```python
from build123d import *

# Parameters (mm, degrees)
F0_R      = 10
F1_DEPTH  = 20
F1_FACE_W = 40
F1_FACE_H = 40
F2_DEPTH  = 10
F4_DEPTH  = 40.001
F5_R      = 4


with BuildPart() as f1:
    # F0 (on Front) → F1 (new body, symmetric)
    with BuildSketch(Plane.XZ):
        Polygon((-12, 21.5), (-20, 21.5), (-20, -21.5), (20, -21.5), (20, 8), align=None)
        Circle(F0_R, mode=Mode.SUBTRACT)
    extrude(amount=F1_DEPTH, both=True)

    # F1_face (on face) → F2 (join)
    with BuildSketch(Plane(origin=(0, 0, -21.5), x_dir=(1, 0, 0), z_dir=(0, 0, -1))):
        Rectangle(F1_FACE_W, F1_FACE_H)
    extrude(amount=F2_DEPTH)

    # F3 (on face) → F4 (cut, through all)
    with BuildSketch(Plane(origin=(-20, 0, 0), x_dir=(0, -1, 0), z_dir=(-1, 0, 0))):
        Polygon((-15, -11.5), (-15, -31.5), (20, -31.5), (20, -16.5), (15, -16.5), (15, -11.5), align=None)
    extrude(amount=-F4_DEPTH, mode=Mode.SUBTRACT)

    # F5
    f5_edges = [f1.edges().sort_by_distance(p)[0] for p in [
        (0, 15, -11.5),
        (0, -15, -11.5),
    ]]
    fillet(f5_edges, radius=F5_R)


solid = f1.part
```
Geometry check sheet. Reference: the model listing, model coordinates, mm. A direction names the side the tool comes from. Coordinates: 2 decimals unless noted, no trailing zeros. Order: outer loops, then holes, each group sorted by start corner. A loop starts at its lowest first (then second) coordinate and runs counter-clockwise, first axis right, second up. Notation, with made-up numbers: (48, 25) - (81, 25) arc R30 cw to (81, 56) - close; hole circle Ø10 at (64, 51.5). An arc over 180 degrees is marked (long way). Answer as a JSON object with one key per item and string values. Group by question number.
Item 1: Draft check along Z on faces 1 (the face through (-2.17, 0.28, -9.76)), 2 (the face through (0, -18, -16.5)), 3 (the face through (-9, -20, -6)), 4 (the face through (4.224, -0.28, 14.656)). Enter one of: +Z half, -Z half, draft (parallel to the pull), parting line (faces both ways), or undercut.
Item 2: Tool access check on faces 5 (the face through (0.28, 13.797, -12.641)), 6 (the face through (20, 0, -3)). Record the directions out of +Z, -Z, +X, -X, +Y, -Y that give a thin tool (end or side, any length) a straight path to the whole face; none if there is none.
Item 3: Sectioned sample at D-D, the plane x = 16. Record the cut outline in (y, z), and give its area (3 significant figures).
Item 4: Sectioned sample at B-B, the plane y = 2. Record the cut outline in (x, z).
Item 5: Depth check by flat-ended pin: pin 1 Ø4 at (x, y) = (-1, 2) entering from +Z; pin 2 Ø17.5 at (x, y) = (-3.5, 1.5) entering from -Z; pin 3 Ø2.5 at (x, y) = (-1.5, -17) entering from -Z. Enter the tip coordinate at first touch or a pass-through.
Item 6: Sectioned sample at A-A, the plane z = 0. Record the cut outline in (x, y), and give its area (3 significant figures).
Item 7: Scan lines: probe 1 along Z at (x, y) = (0, 2); probe 2 along Z at (x, y) = (0, -14.5); probe 3 along Z at (x, y) = (-12, -17). Record each from-to range of solid material in increasing order.
Item 8: Sectioned sample at C-C, the plane x = 0. Record the cut outline in (y, z), and give its area (3 significant figures).
Resolved:
{
 "1": {"face 1": "undercut", "face 2": "-Z half", "face 3": "draft", "face 4": "+Z half"},
 "2": {"face 5": "-Z, +X, -X", "face 6": "+Z, -Z, +X, +Y, -Y"},
 "3": {"outline": "(-20, -16.5) - (-15, -16.5) - (-15, -15.5) arc R4 cw to (-11, -11.5) - (11, -11.5) arc R4 cw to (15, -15.5) - (15, -31.5) - (20, -31.5) - (20, 9.69) - (-20, 9.69) - close", "area": "979 mm^2"},
 "4": {"outline": "(-20, -11.5) - (20, -11.5) - (20, 8) - (-12, 21.5) - (-20, 21.5) - close; hole circle Ø20 at (0, 0)"},
 "5": {"pin 1": "z = 17.7", "pin 2": "z = -11.5", "pin 3": "z = -16.5"},
 "6": {"outline": "(-20, -20) - (-10, -20) - (-10, 20) - (-20, 20) - close; (10, -20) - (20, -20) - (20, 20) - (10, 20) - close", "area": "800 mm^2"},
 "7": {"probe 1": "-11.5 to -10, 10 to 16.44", "probe 2": "-13.56 to -10, 10 to 16.44", "probe 3": "-16.5 to 21.5"},
 "8": {"outline": "(-20, -16.5) - (-15, -16.5) - (-15, -15.5) arc R4 cw to (-11, -11.5) - (11, -11.5) arc R4 cw to (15, -15.5) - (15, -31.5) - (20, -31.5) - (20, -10) - (-20, -10) - close; (-20, 10) - (20, 10) - (20, 16.44) - (-20, 16.44) - close", "area": "449 mm^2"}
}
